from build123d import *

# Parameters (mm, degrees)
PROFILE_R         = 1.15
EXTRUDE_248_DEPTH = 2.6
EXTRUDE_START     = 2.6
PROFILE_2_W       = 6.5
PROFILE_2_H       = 4.4
EXTRUDE_349_DEPTH = 2


with BuildPart() as part:
    # profile → Extrude 248 (new body)
    with BuildSketch(Plane.XY):
        Polygon((25.7, -32), (40.5, -32), (40.5, 3.15), (25.7, 3.15), (25.7, -7.4), (36.4, -7.4), (36.4, -21.6), (25.7, -21.6), align=None)
        with Locations((38.4, -23)):
            Circle(PROFILE_R, mode=Mode.SUBTRACT)
        with Locations((38.4, -0.4)):
            Circle(PROFILE_R, mode=Mode.SUBTRACT)
        with BuildLine():
            Line((28.8, -26.9), (31.4, -26.9))
            ThreePointArc((31.4, -26.9), (32.8, -25.5), (31.4, -24.1))
            Line((31.4, -24.1), (28.8, -24.1))
            ThreePointArc((28.8, -24.1), (27.4, -25.5), (28.8, -26.9))
        make_face(mode=Mode.SUBTRACT)
        with BuildLine():
            Line((28.8, -4.9), (31.4, -4.9))
            ThreePointArc((31.4, -4.9), (32.8, -3.5), (31.4, -2.1))
            Line((31.4, -2.1), (28.8, -2.1))
            ThreePointArc((28.8, -2.1), (27.4, -3.5), (28.8, -4.9))
        make_face(mode=Mode.SUBTRACT)
    extrude(amount=EXTRUDE_248_DEPTH)

    # profile 2 → Extrude 349 (add)
    # profile 1 of 2: a face of its own
    with BuildSketch(Plane.XY.offset(EXTRUDE_START)):
        with Locations((30.15, -25.5)):
            Rectangle(PROFILE_2_W, PROFILE_2_H)
        with BuildLine():
            Line((28.8, -26.9), (31.4, -26.9))
            ThreePointArc((31.4, -26.9), (32.8, -25.5), (31.4, -24.1))
            Line((31.4, -24.1), (28.8, -24.1))
            ThreePointArc((28.8, -24.1), (27.4, -25.5), (28.8, -26.9))
        make_face(mode=Mode.SUBTRACT)
    # profile 2 of 2: a face of its own
    with BuildSketch(Plane.XY.offset(EXTRUDE_START)):
        with Locations((30.15, -3.5)):
            Rectangle(PROFILE_2_W, PROFILE_2_H)
        with BuildLine():
            Line((28.8, -4.9), (31.4, -4.9))
            ThreePointArc((31.4, -4.9), (32.8, -3.5), (31.4, -2.1))
            Line((31.4, -2.1), (28.8, -2.1))
            ThreePointArc((28.8, -2.1), (27.4, -3.5), (28.8, -4.9))
        make_face(mode=Mode.SUBTRACT)
    extrude(amount=EXTRUDE_349_DEPTH)


solid = part.part
Design review of the part built by this model. Coordinates are the model's own, in mm. A direction names the side the tool comes from. Coordinates: 2 decimals unless noted, no trailing zeros. Order: outer loops, then holes, each group sorted by start corner. A loop starts at its lowest first (then second) coordinate and runs counter-clockwise, first axis right, second up. Notation, with made-up numbers: (43, 9) - (99, 9) arc R15 ccw to (99, 25) - close; hole circle Ø8 at (4.25, 77). An arc over 180 degrees is marked (long way). Put each result on its own line as item: value.
1) The part is to be moulded in two halves that separate along X. For faces 1 (the face through (27.4, -3.5, 2.3)), 2 (the face through (30, -4.9, 2)), 3 (the face through (30, -27.7, 4)), 4 (the face through (25.7, -27, 1)), say which applies: released by +X, released by -X, zero draft, split by the parting line, or undercut.
Response values:
face 1: undercut
face 2: undercut
face 3: zero draft
face 4: released by -X
2) Take a section at A-A, the plane x = 29.5. Give the boundary of the cut face in (y, z).
Response values:
outline: (-32, 0) - (-26.9, 0) - (-26.9, 4.6) - (-27.7, 4.6) - (-27.7, 2.6) - (-32, 2.6) - close; (-24.1, 0) - (-21.6, 0) - (-21.6, 2.6) - (-23.3, 2.6) - (-23.3, 4.6) - (-24.1, 4.6) - close; (-7.4, 0) - (-4.9, 0) - (-4.9, 4.6) - (-5.7, 4.6) - (-5.7, 2.6) - (-7.4, 2.6) - close; (-2.1, 0) - (3.15, 0) - (3.15, 2.6) - (-1.3, 2.6) - (-1.3, 4.6) - (-2.1, 4.6) - close
3) Take a section at C-C, the plane y = -0.4. Give the boundary of the cut face in (x, z).
Response values:
outline: (25.7, 0) - (37.25, 0) - (37.25, 2.6) - (25.7, 2.6) - close; (39.55, 0) - (40.5, 0) - (40.5, 2.6) - (39.55, 2.6) - close
4) Tool access review of faces 5 (the face through (26.9, -26, 4)), 6 (the face through (31, -21.6, 1)), 7 (the face through (33, -32, 1)), 8 (the face through (33.4, -4, 4)), 9 (the face through (32.8, -25.5, 2.3)): name each direction out of +Z, -Z, +X, -X, +Y, -Y from which nothing blocks a thin tool from reaching the whole face with its end or side.
Response values:
face 5: +Z, -X, +Y, -Y
face 6: +Z, -Z, -X
face 7: +Z, -Z, +X, -X, -Y
face 8: +Z, +X, +Y, -Y
face 9: +Z, -Z
5) Take a section at B-B, the plane z = 3.35. Give the boundary of the cut face in (x, y), and give its area (3 significant figures).
Response values:
outline: (26.9, -27.7) - (33.4, -27.7) - (33.4, -23.3) - (26.9, -23.3) - close; (26.9, -5.7) - (33.4, -5.7) - (33.4, -1.3) - (26.9, -1.3) - close; hole (28.8, -26.9) - (31.4, -26.9) arc R1.4 ccw to (31.4, -24.1) - (28.8, -24.1) arc R1.4 ccw to start; hole (28.8, -4.9) - (31.4, -4.9) arc R1.4 ccw to (31.4, -2.1) - (28.8, -2.1) arc R1.4 ccw to start
area: 30.3 mm²
6) Insertion check: P1, Ø2, axis at y = -18, z = 1.5, coming from the -X side; P2, Ø0.6, axis at x = 29.5, z = 3.5, coming from the +Y side; P3, Ø0.6, axis at y = -3.5, z = 3.5, coming from the -X side. Each pin has a flat end and moves straight along its axis. Give the tip position at first contact, or say it passes through.
Response values:
P1: stops at x = 36.4
P2: stops at y = -1.3
P3: stops at x = 26.9
7) Take a section at D-D, the plane x = 35. Give the boundary of the cut face in (y, z), and give its area (3 significant figures).
Response values:
outline: (-32, 0) - (-21.6, 0) - (-21.6, 2.6) - (-32, 2.6) - close; (-7.4, 0) - (3.15, 0) - (3.15, 2.6) - (-7.4, 2.6) - close
area: 54.5 mm²
8) Wall thickness on L1, parallel to Y at x = 38.4, z = 1.45; L2, parallel to X at y = -25.5, z = 0.4; L3, parallel to Y at x = 31.25, z = 3.45: over which ranges is each line inside the solid? List them lowest first. Write a range as from..to.
Response values:
L1: y = -32..-24.15, -21.85..-1.55, 0.75..3.15
L2: x = 25.7..27.4, 32.8..40.5
L3: y = -27.7..-26.9, -24.1..-23.3, -5.7..-4.9, -2.1..-1.3
